Verification items for the finished model (mm, model axes). A direction names the side the tool comes from. Give positions to 0.01 mm unless a question says otherwise; leave off trailing zeros. Write each loop counter-clockwise with the first axis right and the second up, starting at its lowest first coordinate (ties: lowest second). Pieces come first, ordered by that corner, then holes. Notation, with made-up numbers: (59.25, 70) -> (90.25, 70) arc R34 ccw to (90.25, 101) -> close; hole circle Ø2 at (-22, -12.5). An arc over 180 degrees is marked (long way). Use one line per item in the form item = value. Start each with the question number.
(1) Release check for a two-part mould opening along Y. For faces 4 (the face through (18.007, 22.404, -58.345)), 5 (the face through (18, 0, -32)), 6 (the face through (-17.5, 16, -32)) record: pulls with the +Y half, pulls with the -Y half, needs draft (parallel to the pull), parting line crosses it, or undercut.
(2) Set-up check for faces 1 (the face through (-18.01, 16.7, -42.63)), 2 (the face through (4, 12, 0)), 3 (the face through (18.007, 20.433, -7.159)): record each of +Z, -Z, +X, -X, +Y, -Y from which the full face is reachable in a straight line by a thin tool's end or side.
(3) Section check C-C, the plane x = -10.5. Record the cut outline in (y, z), plus the area to 3 significant figures.
(4) Depth check by flat-ended pin: pin 1 Ø9.5 at (y, z) = (13, -26) entering from +X; pin 2 Ø8 at (y, z) = (25, -46.5) entering from +X; pin 3 Ø1.6 at (x, y) = (-5.72, 10.28) entering from -Z; pin 4 Ø0.5 at (x, y) = (18, 18) entering from +Z. Enter the tip coordinate at first touch or a pass-through.
(5) Section check A-A, the plane z = -52. Record the cut outline in (x, y).
(6) Section check B-B, the plane y = 27.5. Record the cut outline in (x, z), plus the area to 3 significant figures.
(7) Scan lines: L1, parallel to Y at x = 8, z = 0.2; L2, parallel to X at y = 7, z = -6; L3, parallel to X at y = 20, z = -34. Record each from-to range of solid material in increasing order.
from build123d import *

# Parameters (mm, degrees)
EXTRUDE_THIN2_DEPTH = 32
FILLET4_R           = 1
FILLET5_R           = 1
FILLET6_R           = 1
FILLET7_R           = 1
FILLET8_R           = 1
FILLET9_R           = 1
SKETCH9_W           = 42.294810508
SKETCH9_H           = 21
CUT_EXTRUDE2_DEPTH  = 32
SKETCH10_R          = 5
CUT_EXTRUDE3_DEPTH  = 32
SKETCH14_R          = 0.6
CUT_EXTRUDE7_DEPTH  = 32
SKETCH15_R          = 0.6
CUT_EXTRUDE8_DEPTH  = 10
SKETCH13_R          = 2.535991587
CUT_EXTRUDE9_DEPTH  = 10
SKETCH11_R          = 2.032571361
SKETCH11_R_2        = 2.028056202
CUT_EXTRUDE12_DEPTH = 10
SKETCH16_R          = 2
CUT_EXTRUDE13_DEPTH = 10


with BuildPart() as part:
    # Sketch8 → Extrude-Thin2 (new body)
    with BuildSketch(Plane(origin=(0, 0, 0), x_dir=(1, 0, 0), z_dir=(0, 1, 0))):
        Polygon((17.5, 65), (17.5, 0), (-17.5, 0), (-17.5, 65), (-18.5, 65), (-18.5, -1), (18.5, -1), (18.5, 65), align=None)
    extrude(amount=EXTRUDE_THIN2_DEPTH)

    # Fillet4
    fillet4_edges = [part.edges().sort_by_distance(p)[0] for p in [
        (-18, 0, -65),
    ]]
    fillet(fillet4_edges, radius=FILLET4_R)

    # Fillet5
    fillet5_edges = [part.edges().sort_by_distance(p)[0] for p in [
        (-18, 32, -65),
    ]]
    fillet(fillet5_edges, radius=FILLET5_R)

    # Fillet6
    fillet6_edges = [part.edges().sort_by_distance(p)[0] for p in [
        (18, 0, -65),
    ]]
    fillet(fillet6_edges, radius=FILLET6_R)

    # Fillet7
    fillet7_edges = [part.edges().sort_by_distance(p)[0] for p in [
        (18, 32, -65),
    ]]
    fillet(fillet7_edges, radius=FILLET7_R)

    # Fillet8
    fillet8_edges = [part.edges().sort_by_distance(p)[0] for p in [
        (18.5, 16, 1),
    ]]
    fillet(fillet8_edges, radius=FILLET8_R)

    # Fillet9
    fillet9_edges = [part.edges().sort_by_distance(p)[0] for p in [
        (-18.5, 16, 1),
    ]]
    fillet(fillet9_edges, radius=FILLET9_R)

    # Sketch9 → Cut-Extrude2 (cut)
    with BuildSketch(Plane(origin=(18.5, 0, 0), x_dir=(0, 0, -1), z_dir=(1, 0, 0))):
        with Locations((32, 16)):
            Rectangle(SKETCH9_W, SKETCH9_H)
    extrude(amount=-CUT_EXTRUDE2_DEPTH, mode=Mode.SUBTRACT)

    # Sketch10 → Cut-Extrude3 (cut)
    with BuildSketch(Plane.XY.offset(1)):
        with Locations((0, 16)):
            Circle(SKETCH10_R)
    extrude(amount=-CUT_EXTRUDE3_DEPTH, mode=Mode.SUBTRACT)

    # Sketch14 → Cut-Extrude7 (cut)
    with BuildSketch(Plane.XY.offset(1)):
        with Locations((0, 7.914892415)):
            Circle(SKETCH14_R)
        with Locations((0, 24.085107585)):
            Circle(SKETCH14_R)
        with Locations((-5.7170344, 10.2829656)):
            Circle(SKETCH14_R)
        with Locations((-5.7170344, 21.7170344)):
            Circle(SKETCH14_R)
        with Locations((5.7170344, 10.2829656)):
            Circle(SKETCH14_R)
        with Locations((5.7170344, 21.7170344)):
            Circle(SKETCH14_R)
    extrude(amount=-CUT_EXTRUDE7_DEPTH, mode=Mode.SUBTRACT)

    # Sketch15 → Cut-Extrude8 (cut)
    with BuildSketch(Plane.XY.offset(1)):
        with Locations((-8, 16)):
            Circle(SKETCH15_R)
        with Locations((8, 16)):
            Circle(SKETCH15_R)
    extrude(amount=-CUT_EXTRUDE8_DEPTH, mode=Mode.SUBTRACT)

    # Sketch13 → Cut-Extrude9 (cut)
    with BuildSketch(Plane.ZY.offset(18.5)):
        with Locations((-45.049639152, 15.939767339)):
            Circle(SKETCH13_R)
    extrude(amount=-CUT_EXTRUDE9_DEPTH, mode=Mode.SUBTRACT)

    # Sketch11 → Cut-Extrude12 (cut)
    with BuildSketch(Plane(origin=(18.5, 0, 0), x_dir=(0, 0, -1), z_dir=(1, 0, 0))):
        with Locations((56.406137915, 21.793575716)):
            Circle(SKETCH11_R)
        with Locations((56.406137915, 10.115569331)):
            Circle(SKETCH11_R_2)
    extrude(amount=-CUT_EXTRUDE12_DEPTH, mode=Mode.SUBTRACT)

    # Sketch16 → Cut-Extrude13 (cut)
    with BuildSketch(Plane(origin=(18.5, 0, 0), x_dir=(0, 0, -1), z_dir=(1, 0, 0))):
        with Locations((7.592594746, 22.385297204)):
            Circle(SKETCH16_R)
        with Locations((7.592594746, 10.115569331)):
            Circle(SKETCH16_R)
    extrude(amount=-CUT_EXTRUDE13_DEPTH, mode=Mode.SUBTRACT)


solid = part.part
Completed:
q1.face_4 = undercut
q1.face_5 = pulls with the -Y half
q1.face_6 = needs draft
q2.face_1 = +X, -X
q2.face_2 = -Z, +Y, -Y
q2.face_3 = +X
q3.outline = (0, 0) -> (32, 0) -> (32, 1) -> (0, 1) -> close
q3.area = 32.0 mm²
q4.pin_1 = -17.5
q4.pin_2 = 18.5
q4.pin_3 = 0
q4.pin_4 = 0.97
q5.outline = (-18.5, 0) -> (-17.5, 0) -> (-17.5, 32) -> (-18.5, 32) -> close; (17.5, 0) -> (18.5, 0) -> (18.5, 5.5) -> (17.5, 5.5) -> close; (17.5, 26.5) -> (18.5, 26.5) -> (18.5, 32) -> (17.5, 32) -> close
q6.outline = (-18.5, -65) -> (-17.5, -65) -> (-17.5, 0) -> (17.5, 0) -> (17.5, -65) -> (18.5, -65) -> (18.5, 0) arc R1 ccw to (17.5, 1) -> (-17.5, 1) arc R1 ccw to (-18.5, 0) -> close
q6.area = 167 mm²
q7.L1 = 0 to 15.4, 16.6 to 32
q7.L2 = -18.5 to -17.5, 17.5 to 18.5
q7.L3 = -18.5 to -17.5
